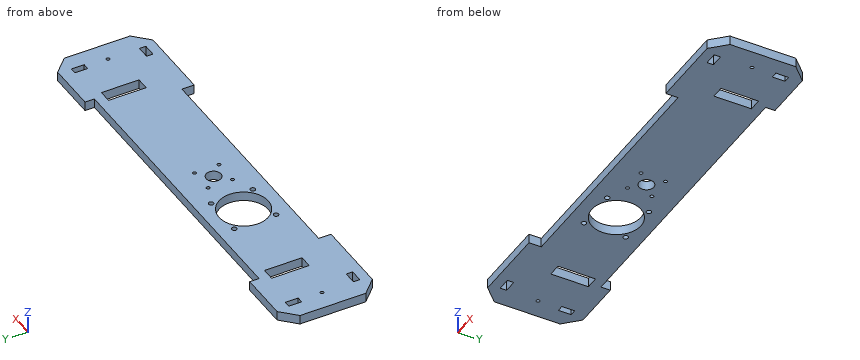
```python
from build123d import *

# Parameters (mm, degrees)
CROQUIS1_R              = 3.5
CROQUIS1_R_2            = 15
CROQUIS1_R_3            = 50
CROQUIS1_R_4            = 5
CROQUIS1_W              = 26
CROQUIS1_H              = 76.5
CROQUIS1_H_2            = 13
CROQUIS1_W_2            = 13
CROQUIS1_H_3            = 26
SALIENTE_EXTRUIR1_DEPTH = 19


with BuildPart() as part:
    # Croquis1 → Saliente-Extruir1 (new body)
    with BuildSketch(Plane.XY):
        Polygon((-301, 194), (-301, 175), (301, 175), (301, 194), (401, 194), (431, 164), (431, 30), (401, 0), (250, 0), (250, 25), (-250, 25), (-250, 0), (-401, 0), (-431, 30), (-431, 164), (-401, 194), align=None)
        with Locations((-391, 97)):
            Circle(CROQUIS1_R, mode=Mode.SUBTRACT)
        with Locations((391, 97)):
            Circle(CROQUIS1_R, mode=Mode.SUBTRACT)
        with Locations((0, 100)):
            Circle(CROQUIS1_R_2, mode=Mode.SUBTRACT)
        with Locations((-25, 125)):
            Circle(CROQUIS1_R, mode=Mode.SUBTRACT)
        with Locations((25, 125)):
            Circle(CROQUIS1_R, mode=Mode.SUBTRACT)
        with Locations((25, 75)):
            Circle(CROQUIS1_R, mode=Mode.SUBTRACT)
        with Locations((-25, 75)):
            Circle(CROQUIS1_R, mode=Mode.SUBTRACT)
        with Locations((-110, 100)):
            Circle(CROQUIS1_R_3, mode=Mode.SUBTRACT)
        with Locations((-152.426406871, 142.426406871)):
            Circle(CROQUIS1_R_4, mode=Mode.SUBTRACT)
        with Locations((-67.573593129, 142.426406871)):
            Circle(CROQUIS1_R_4, mode=Mode.SUBTRACT)
        with Locations((-67.573593129, 57.573593129)):
            Circle(CROQUIS1_R_4, mode=Mode.SUBTRACT)
        with Locations((-152.426406871, 57.573593129)):
            Circle(CROQUIS1_R_4, mode=Mode.SUBTRACT)
        with Locations((-298, 116.75)):
            Rectangle(CROQUIS1_W, CROQUIS1_H, mode=Mode.SUBTRACT)
        with Locations((298, 116.75)):
            Rectangle(CROQUIS1_W, CROQUIS1_H, mode=Mode.SUBTRACT)
        with Locations((378, 26.5)):
            Rectangle(CROQUIS1_W, CROQUIS1_H_2, mode=Mode.SUBTRACT)
        with Locations((-378, 26.5)):
            Rectangle(CROQUIS1_W, CROQUIS1_H_2, mode=Mode.SUBTRACT)
        with Locations((391, 155)):
            Rectangle(CROQUIS1_W_2, CROQUIS1_H_3, mode=Mode.SUBTRACT)
        with Locations((-391, 155)):
            Rectangle(CROQUIS1_W_2, CROQUIS1_H_3, mode=Mode.SUBTRACT)
    extrude(amount=SALIENTE_EXTRUIR1_DEPTH)


solid = part.part
```
Source: CAD feature listing. Evaluate the final solid. Frame: model axes, mm. Give positions to 0.01 mm unless a question says otherwise; leave off trailing zeros. Loops run counter-clockwise (first coordinate to the right, second up) from the corner with the lowest first, then second, coordinate; pieces in that order, holes last. Notation, with made-up numbers: (-18, 76) - (-5, 76) arc R37 cw to (-5, 113) - close; hole circle Ø3 at (15.5, 59.25). An arc over 180 degrees is marked (long way). Use CSV: the item, a comma, the result in double quotes.
1) Cut plane B-B (x = 84.5). Output: boundary loops of the cut face in (y, z).
Worked out:
outline,"(25, 0) - (175, 0) - (175, 19) - (25, 19) - close"
2) Cut plane C-C (z = 13.5). Count the separate pieces of the cut face and the enclosed holes in it, and give its area (3 significant figures).
Worked out:
separate pieces,"1"
enclosed holes,"18"
area,"127,000 mm^2"
3) Pin query (flat end, axial travel): P1, Ø9.5, axis at y = 17, z = 13, coming from the -X side; P2, Ø4, axis at y = 26, z = 11.5, coming from the -X side; P3, Ø3, axis at x = 308, y = 83.5, coming from the +Z side; P4, Ø13, axis at x = -67.57, y = 142.43, coming from the -Z side. Return the tip coordinate at first contact, or that it passes through.
Worked out:
P1,"stops at x = -422.75"
P2,"stops at x = -429"
P3,"passes through"
P4,"stops at z = 0"
4) Line query: line 1 (Y direction, x = -25, z = 7.75); line 2 (X direction, y = 164, z = 8.5); line 3 (X direction, y = 110.5, z = 15.75). Output: solid intervals per line, ascending.
Worked out:
line 1,"y = 25 to 71.5, 78.5 to 121.5, 128.5 to 175"
line 2,"x = -431 to -397.5, -384.5 to 384.5, 397.5 to 431"
line 3,"x = -431 to -311, -285 to -158.89, -61.11 to -10.71, 10.71 to 285, 311 to 431"
5) Cut plane A-A (x = -110). Output: boundary loops of the cut face in (y, z).
Worked out:
outline,"(25, 0) - (50, 0) - (50, 19) - (25, 19) - close; (150, 0) - (175, 0) - (175, 19) - (150, 19) - close"
